Here's how the part is built. I have some questions about the finished solid (model axes, mm). A direction names the side the tool comes from. Round coordinates to 2 decimals unless told otherwise and drop trailing zeros. Order: outer loops, then holes, each group sorted by start corner. A loop starts at its lowest first (then second) coordinate and runs counter-clockwise, first axis right, second up. Notation, with made-up numbers: (30.25, 13.5) - (51.25, 13.5) arc R19 ccw to (51.25, 36.5) - close; hole circle Ø10 at (-40, 23.25). An arc over 180 degrees is marked (long way). Answer as a JSON object with one key per item and string values.
Autodesk Inventor part; units mm, degrees
ref_plane "YZ Plane" through (0, 0, 0) normal (1, 0, 0) x (0, 1, 0)
ref_plane "XZ Plane" through (0, 0, 0) normal (0, 1, 0) x (-1, 0, 0)
ref_plane "XY Plane" through (0, 0, 0) normal (0, 0, 1) x (1, 0, 0)
sketch "Sketch1" plane through (0, 0, 0) normal (0, 1, 0) x (-1, 0, 0)
  line L0 (-38.1, 9.525) -> (38.1, 9.525)
  line L1 (38.1, 9.525) -> (38.1, -9.525)
  line L2 (38.1, -9.525) -> (-38.1, -9.525)
  line L3 (-38.1, -9.525) -> (-38.1, 9.525)
  line L4 (-38.1, 9.525) -> (38.1, -9.525) construction
  line L5 (38.1, 9.525) -> (-38.1, -9.525) construction
  point P0 (0, 0)
  dimension "d0" = 76.2
  dimension "d1" = 19.05
extrude "Extrusion1" add sketch "Sketch1" along normal mid plane 12.7
sketch "Sketch2" plane through (38.1, -6.35, -9.525) normal (1, 0, 0) x (0, 0, -1)
  line L0 (0, 3.663) -> (-2.687, 6.35)
  line L1 (-2.687, 6.35) -> (0, 9.037)
  line L2 (0, 9.037) -> (2.687, 6.35)
  line L3 (2.687, 6.35) -> (0, 3.663)
  line L4 (-19.05, 12.7) -> (0, 12.7)
  line L5 (0, 12.7) -> (0, 0)
  point P0 (-9.525, 6.35)
  point P1 (0, 6.35)
  dimension "d4" = 45
  dimension "d5" = 3.8
extrude "Extrusion2" cut sketch "Sketch2" against normal through all
sketch "Sketch5" plane through (0, 6.35, 0) normal (0, 1, 0) x (1, 0, 0)
  line L0 (-38.1, 9.525) -> (-38.1, -9.525)
  line L1 (38.1, -9.525) -> (38.1, 9.525)
  point P0 (0, 0)
  point P1 (-25.4, 0)
  point P2 (25.4, 0)
  dimension "d18" = 12.7
  dimension "d19" = 12.7
hole "Hole1" at (-25.4, 6.35, 0) at (25.4, 6.35, 0) direction (0, -1, 0) diameter 5.3086 end through all
sketch "Sketch7" plane through (0, 6.35, 0) normal (0, 1, 0) x (1, 0, 0)
  circle A0 centre (-25.4, 0) radius 2.6543
  circle A1 centre (25.4, 0) radius 2.6543
  line L0 (-23.004, 4.15) -> (-20.608, 0)
  line L1 (-20.608, 0) -> (-23.004, -4.15)
  line L2 (-23.004, -4.15) -> (-27.796, -4.15)
  line L3 (-27.796, -4.15) -> (-30.192, 0)
  line L4 (-30.192, 0) -> (-27.796, 4.15)
  line L5 (-27.796, 4.15) -> (-23.004, 4.15)
  line L6 (23.004, -4.15) -> (20.608, 0)
  line L7 (20.608, 0) -> (23.004, 4.15)
  line L8 (23.004, 4.15) -> (27.796, 4.15)
  line L9 (27.796, 4.15) -> (30.192, 0)
  line L10 (30.192, 0) -> (27.796, -4.15)
  line L11 (27.796, -4.15) -> (23.004, -4.15)
  point P0 (0, 0)
  dimension "d39" = 8.3
  dimension "d40" = 8.3
extrude "Extrusion5" cut sketch "Sketch7" against normal blind 4.7625 contours A1 | L0 L1 L2 L3 L4 L5 | L6 L7 L8 L9 L10 L11
sketch "Sketch8" plane through (0, 6.35, 0) normal (0, 1, 0) x (1, 0, 0)
  point P0 (0, 0)
  point P1 (-7, -5)
  point P2 (-7, 5)
  dimension "d43" = 10
  dimension "d52" = 7
  dimension "d53" = 5
hole "Hole3" at (-7, 6.35, 5) at (-7, 6.35, -5) direction (0, -1, 0) diameter 2.459 depth 8.7884
equation "\"d40\" = d39"
properties part number "X-Axis_Mount_Slide_Endstop_MountLM3046" material "Acetal Resin, White"
1. If I drill on L1, parallel to X at y = -3, z = 0; L2, parallel to X at y = 0, z = 5; L3, parallel to X at y = 5.25, z = 3.25, over which ranges is the centre line in solid material (lowest first)? Write a range as [from, to].
Responses:
{"L1": "[-38.1, -28.05], [-22.75, 22.75], [28.05, 38.1]", "L2": "[-38.1, -8.23], [-5.77, 38.1]", "L3": "[-38.1, -28.32], [-22.48, 22.48], [28.32, 38.1]"}
2. Thinking about a two-plate mould opening in X: for faces 1 (the face through (-1, -5, -9.525)), 2 (the face through (38.1, 0, 0)), 3 (the face through (21.82, 4, 2.1)), which applies, pulls with the +X half, pulls with the -X half, needs draft (parallel to the pull), parting line crosses it, or undercut?
Responses:
{"face 1": "needs draft", "face 2": "pulls with the +X half", "face 3": "undercut"}
3. Imagine slicing it at C-C (y = 0.75). List the corners of the cut face in (x, z) for me (1 decimal), plus the area to 3 significant figures.
Responses:
{"outline": "(-38.1, -7.6) - (38.1, -7.6) - (38.1, 9.5) - (-38.1, 9.5) - close; hole circle Ø5.3 at (-25.4, 0); hole circle Ø2.5 at (-7, -5); hole circle Ø2.5 at (-7, 5); hole circle Ø5.3 at (25.4, 0)", "area": "1,250 mm2"}
4. Imagine slicing it at B-B (z = 0.75). List the corners of the cut face in (x, y) for me, plus the area to 3 significant figures.
Responses:
{"outline": "(-38.1, -6.35) - (-27.95, -6.35) - (-27.95, 1.59) - (-29.76, 1.59) - (-29.76, 6.35) - (-38.1, 6.35) - close; (-22.85, -6.35) - (22.85, -6.35) - (22.85, 1.59) - (21.04, 1.59) - (21.04, 6.35) - (-21.04, 6.35) - (-21.04, 1.59) - (-22.85, 1.59) - close; (27.95, -6.35) - (38.1, -6.35) - (38.1, 6.35) - (29.76, 6.35) - (29.76, 1.59) - (27.95, 1.59) - close", "area": "804 mm2"}
5. For P1, Ø6, axis at x = 25.4, z = 0, coming from the +Y side; P2, Ø2, axis at x = -7, z = 5, coming from the +Y side, each with a flat end and sliding along its axis, tell me the tip position at first contact or that it passes through.
Responses:
{"P1": "y = 1.59", "P2": "y = -2.44"}
6. Imagine slicing it at D-D (z = -8). List the corners of the cut face in (x, y) for me.
Responses:
{"outline": "(-38.1, -6.35) - (38.1, -6.35) - (38.1, -1.16) - (-38.1, -1.16) - close; (-38.1, 1.16) - (38.1, 1.16) - (38.1, 6.35) - (-38.1, 6.35) - close"}
7. For faces 4 (the face through (0.53, 1.32, -8.16)), 5 (the face through (-25, 4, 4.15)), 6 (the face through (1, -6.35, 0)), which set-ups out of +Z, -Z, +X, -X, +Y, -Y let a thin tool reach every point of the face, with its end or its side?
Responses:
{"face 4": "-Z, +X, -X", "face 5": "+Y", "face 6": "+Z, -Z, +X, -X, -Y"}
